from build123d import *

# Parameters (mm, degrees)
ESBO_O1_R                = 32
RESSALTO_EXTRUS_O4_DEPTH = 6
ESBO_O2_R                = 2
CORTE_EXTRUS_O1_DEPTH    = 6


with BuildPart() as part:
    # Esboço1 → Ressalto-extrusão4 (new body)
    with BuildSketch(Plane.XY):
        Circle(ESBO_O1_R)
        with BuildLine():
            Line((-2.646462789, 26.86998762), (-2.450428508, 24.879618167))
            ThreePointArc((-2.450428508, 24.879618167), (-4.87725805, 24.51963201), (-7.257116931, 23.923508393))
            Line((-7.257116931, 23.923508393), (-7.837686286, 25.837389065))
            ThreePointArc((-7.837686286, 25.837389065), (-9.096026042, 25.42168976), (-10.332452674, 24.944747378))
            ThreePointArc((-10.332452674, 24.944747378), (-11.543987523, 24.407710914), (-12.727711894, 23.811874137))
            Line((-12.727711894, 23.811874137), (-11.784918421, 22.048031609))
            ThreePointArc((-11.784918421, 22.048031609), (-13.889255825, 20.786740308), (-15.859832104, 19.325261334))
            Line((-15.859832104, 19.325261334), (-17.128618672, 20.871282241))
            ThreePointArc((-17.128618672, 20.871282241), (-18.132091781, 20.005680385), (-19.091883092, 19.091883092))
            ThreePointArc((-19.091883092, 19.091883092), (-20.005680385, 18.132091781), (-20.871282241, 17.128618672))
            Line((-20.871282241, 17.128618672), (-19.325261334, 15.859832104))
            ThreePointArc((-19.325261334, 15.859832104), (-20.786740308, 13.889255825), (-22.048031609, 11.784918421))
            Line((-22.048031609, 11.784918421), (-23.811874137, 12.727711894))
            ThreePointArc((-23.811874137, 12.727711894), (-24.407710914, 11.543987523), (-24.944747378, 10.332452674))
            ThreePointArc((-24.944747378, 10.332452674), (-25.42168976, 9.096026042), (-25.837389065, 7.837686286))
            Line((-25.837389065, 7.837686286), (-23.923508393, 7.257116931))
            ThreePointArc((-23.923508393, 7.257116931), (-24.51963201, 4.87725805), (-24.879618167, 2.450428508))
            Line((-24.879618167, 2.450428508), (-26.86998762, 2.646462789))
            ThreePointArc((-26.86998762, 2.646462789), (-26.967477318, 1.324827207), (-27, 0))
            ThreePointArc((-27, 0), (-26.967477318, -1.324827207), (-26.86998762, -2.646462789))
            Line((-26.86998762, -2.646462789), (-24.879618167, -2.450428508))
            ThreePointArc((-24.879618167, -2.450428508), (-24.51963201, -4.87725805), (-23.923508393, -7.257116931))
            Line((-23.923508393, -7.257116931), (-25.837389065, -7.837686286))
            ThreePointArc((-25.837389065, -7.837686286), (-25.42168976, -9.096026042), (-24.944747378, -10.332452674))
            ThreePointArc((-24.944747378, -10.332452674), (-24.407710914, -11.543987523), (-23.811874137, -12.727711894))
            Line((-23.811874137, -12.727711894), (-22.048031609, -11.784918421))
            ThreePointArc((-22.048031609, -11.784918421), (-20.786740308, -13.889255825), (-19.325261334, -15.859832104))
            Line((-19.325261334, -15.859832104), (-20.871282241, -17.128618672))
            ThreePointArc((-20.871282241, -17.128618672), (-20.005680385, -18.132091781), (-19.091883092, -19.091883092))
            ThreePointArc((-19.091883092, -19.091883092), (-18.132091781, -20.005680385), (-17.128618672, -20.871282241))
            Line((-17.128618672, -20.871282241), (-15.859832104, -19.325261334))
            ThreePointArc((-15.859832104, -19.325261334), (-13.889255825, -20.786740308), (-11.784918421, -22.048031609))
            Line((-11.784918421, -22.048031609), (-12.727711894, -23.811874137))
            ThreePointArc((-12.727711894, -23.811874137), (-11.543987523, -24.407710914), (-10.332452674, -24.944747378))
            ThreePointArc((-10.332452674, -24.944747378), (-9.096026042, -25.42168976), (-7.837686286, -25.837389065))
            Line((-7.837686286, -25.837389065), (-7.257116931, -23.923508393))
            ThreePointArc((-7.257116931, -23.923508393), (-4.87725805, -24.51963201), (-2.450428508, -24.879618167))
            Line((-2.450428508, -24.879618167), (-2.646462789, -26.86998762))
            ThreePointArc((-2.646462789, -26.86998762), (-1.324827207, -26.967477318), (0, -27))
            ThreePointArc((0, -27), (1.324827207, -26.967477318), (2.646462789, -26.86998762))
            Line((2.646462789, -26.86998762), (2.450428508, -24.879618167))
            ThreePointArc((2.450428508, -24.879618167), (4.87725805, -24.51963201), (7.257116931, -23.923508393))
            Line((7.257116931, -23.923508393), (7.837686286, -25.837389065))
            ThreePointArc((7.837686286, -25.837389065), (9.096026042, -25.42168976), (10.332452674, -24.944747378))
            ThreePointArc((10.332452674, -24.944747378), (11.543987523, -24.407710914), (12.727711894, -23.811874137))
            Line((12.727711894, -23.811874137), (11.784918421, -22.048031609))
            ThreePointArc((11.784918421, -22.048031609), (13.889255825, -20.786740308), (15.859832104, -19.325261334))
            Line((15.859832104, -19.325261334), (17.128618672, -20.871282241))
            ThreePointArc((17.128618672, -20.871282241), (18.132091781, -20.005680385), (19.091883092, -19.091883092))
            ThreePointArc((19.091883092, -19.091883092), (20.005680385, -18.132091781), (20.871282241, -17.128618672))
            Line((20.871282241, -17.128618672), (19.325261334, -15.859832104))
            ThreePointArc((19.325261334, -15.859832104), (20.786740308, -13.889255825), (22.048031609, -11.784918421))
            Line((22.048031609, -11.784918421), (23.811874137, -12.727711894))
            ThreePointArc((23.811874137, -12.727711894), (24.407710914, -11.543987523), (24.944747378, -10.332452674))
            ThreePointArc((24.944747378, -10.332452674), (25.42168976, -9.096026042), (25.837389065, -7.837686286))
            Line((25.837389065, -7.837686286), (23.923508393, -7.257116931))
            ThreePointArc((23.923508393, -7.257116931), (24.51963201, -4.87725805), (24.879618167, -2.450428508))
            Line((24.879618167, -2.450428508), (26.86998762, -2.646462789))
            ThreePointArc((26.86998762, -2.646462789), (26.967477318, -1.324827207), (27, 0))
            ThreePointArc((27, 0), (26.967477318, 1.324827207), (26.86998762, 2.646462789))
            Line((26.86998762, 2.646462789), (24.879618167, 2.450428508))
            ThreePointArc((24.879618167, 2.450428508), (24.51963201, 4.87725805), (23.923508393, 7.257116931))
            Line((23.923508393, 7.257116931), (25.837389065, 7.837686286))
            ThreePointArc((25.837389065, 7.837686286), (25.42168976, 9.096026042), (24.944747378, 10.332452674))
            ThreePointArc((24.944747378, 10.332452674), (24.407710914, 11.543987523), (23.811874137, 12.727711894))
            Line((23.811874137, 12.727711894), (22.048031609, 11.784918421))
            ThreePointArc((22.048031609, 11.784918421), (20.786740308, 13.889255825), (19.325261334, 15.859832104))
            Line((19.325261334, 15.859832104), (20.871282241, 17.128618672))
            ThreePointArc((20.871282241, 17.128618672), (20.005680385, 18.132091781), (19.091883092, 19.091883092))
            ThreePointArc((19.091883092, 19.091883092), (18.132091781, 20.005680385), (17.128618672, 20.871282241))
            Line((17.128618672, 20.871282241), (15.859832104, 19.325261334))
            ThreePointArc((15.859832104, 19.325261334), (13.889255825, 20.786740308), (11.784918421, 22.048031609))
            Line((11.784918421, 22.048031609), (12.727711894, 23.811874137))
            ThreePointArc((12.727711894, 23.811874137), (11.543987523, 24.407710914), (10.332452674, 24.944747378))
            ThreePointArc((10.332452674, 24.944747378), (9.096026042, 25.42168976), (7.837686286, 25.837389065))
            Line((7.837686286, 25.837389065), (7.257116931, 23.923508393))
            ThreePointArc((7.257116931, 23.923508393), (4.87725805, 24.51963201), (2.450428508, 24.879618167))
            Line((2.450428508, 24.879618167), (2.646462789, 26.86998762))
            ThreePointArc((2.646462789, 26.86998762), (1.324827207, 26.967477318), (0, 27))
            ThreePointArc((0, 27), (-1.324827207, 26.967477318), (-2.646462789, 26.86998762))
        make_face(mode=Mode.SUBTRACT)
    extrude(amount=RESSALTO_EXTRUS_O4_DEPTH)

    # Esboço2 → Corte-extrusão1 (cut)
    with BuildSketch(Plane.XY.offset(6)):
        with Locations((-5.560074177, 27.952380491)):
            Circle(ESBO_O2_R)
        with Locations((5.560074177, -27.952380491)):
            Circle(ESBO_O2_R)
        with Locations((27.952380491, 5.560074177)):
            Circle(ESBO_O2_R)
        with Locations((-27.952380491, -5.560074177)):
            Circle(ESBO_O2_R)
    extrude(amount=-CORTE_EXTRUS_O1_DEPTH, mode=Mode.SUBTRACT)


solid = part.part
Verification items for the finished model (mm, model axes). Give positions to 0.01 mm unless a question says otherwise; leave off trailing zeros. Write each loop counter-clockwise with the first axis right and the second up, starting at its lowest first coordinate (ties: lowest second). Pieces come first, ordered by that corner, then holes.
(1) Cross-section at B-B (z = 4.05). State how many separate pieces and enclosed holes the cut face has, plus the area to 3 significant figures.
(2) Gauge pin test, flat ends, axial feed: pin 1 (2.5 mm diameter, centred on x = -27.95, y = -5.56, fed in from +Z); pin 2 (2 mm diameter, centred on x = -3, z = 4, fed in from +Y); pin 3 (1 mm diameter, centred on y = 21.5, z = 1.5, fed in from +X). Record the tip position at first contact, or that the pin passes through.
(3) Cross-section at A-A (y = -1). Enter the section's corners in (x, z), plus the area to 3 significant figures.
(4) Mould release check, pull along Y, two halves, no side actions. Record for faces 1 (the face through (2.547, 25.861, 2.958)), 2 (the face through (-14, -21, 0)), 3 (the face through (-6.94, -31.24, 2.96)): +Y half, -Y half, draft (parallel to the pull), parting line (faces both ways), or undercut.
(5) Material ranges on line 1 (X direction, y = -20.5, z = 1.6); line 2 (X direction, y = 19.5, z = 5.4), recorded low to high.
Worked out:
1. separate pieces: 1
1. enclosed holes: 5
1. area: 1,040 mm2
2. pin 1: passes through
2. pin 2: stops at y = 31.94
2. pin 3: stops at x = 24.15
3. outline: (-31.98, 0) - (-26.98, 0) - (-26.98, 6) - (-31.98, 6) - close; (26.98, 0) - (31.98, 0) - (31.98, 6) - (26.98, 6) - close
3. area: 60.0 mm2
4. face 1: undercut
4. face 2: draft
4. face 3: parting line
5. line 1: x = -24.57 to -17.57, -16.82 to -14.31, 14.31 to 16.82, 17.57 to 24.57
5. line 2: x = -25.37 to -18.67, -16 to -15.64, 15.64 to 16, 18.67 to 25.37
